Could you check a few things on this model? Use its own coordinates, in mm. A direction names the side the tool comes from. Coordinates: 2 decimals unless noted, no trailing zeros. Order: outer loops, then holes, each group sorted by start corner. A loop starts at its lowest first (then second) coordinate and runs counter-clockwise, first axis right, second up. Notation, with made-up numbers: (-28, 23) - (22, 23) arc R26 cw to (22, 47) - close; hole circle Ø3 at (-34.75, 14.25). An arc over 180 degrees is marked (long way). Answer as a JSON object with one key per item and string values. Group by question number.
(1) Imagine slicing it at D-D, the plane y = 0. Write out the boundary of the cut face in (x, z), and give its area (3 significant figures).
(2) Please list where these lines run through material, in increasing order: probe 1 along X at (y, z) = (0, 1.5); probe 2 along Y at (x, z) = (0, 8.8); probe 3 along Y at (x, z) = (0, 5.75).
(3) Which directions (+Z, -Z, +X, -X, +Y, -Y) give clear straight access to the entire face, cutting with the end or side of a thin tool? Please do faces 1 (the cylindrical face through (14, 0, 3)), 2 (the flat face through (-17.48, -3.77, 1.6)), 3 (the cylindrical face through (-14.99, 4.58, 6.12)).
(4) Imagine slicing it at A-A, the plane x = 0. Write out the boundary of the cut face in (y, z).
(5) Imagine slicing it at C-C, the plane z = 4.5. Write out the boundary of the cut face in (x, y).
(6) We'd pull the mould along X, two halves only. Please class faces 4 (the flat face through (0, 4.5, 4)), 5 (the flat face through (1, 4, 9)), 6 (the flat face through (17.48, -3.77, 1.55)): pulls with the +X half, pulls with the -X half, needs draft (parallel to the pull), parting line crosses it, or undercut.
(7) Will these pins go through, and if not, where does the flat tip stop? P1, Ø3.5, axis at x = 0, y = 0, coming from the -Z side; P2, Ø5, axis at x = -9, y = 9, coming from the -Z side; P3, Ø0.9, axis at y = 0.5, z = 2, coming from the +X side; P4, Ø9.5, axis at x = -32.5, y = 5, coming from the -Z side.
(8) Imagine slicing it at B-B, the plane z = 0.75. Write out the boundary of the cut face in (x, y).
from build123d import *

# Parameters (mm, degrees)
SKETCH1_W                    = 77.5
SKETCH1_H                    = 7
BOSS_EXTRUDE1_DEPTH          = 9
BOSS_EXTRUDE1_DEPTH_BACK     = 9
SKETCH2_W                    = 20
SKETCH2_H                    = 6.3
CUT_EXTRUDE1_DEPTH           = 8
SKETCH3_W                    = 12.5
SKETCH3_H                    = 5.85
BOSS_EXTRUDE2_DEPTH          = 8
SKETCH4_R                    = 3.04
CUT_EXTRUDE2_DEPTH           = 22
CUT_EXTRUDE2_DEPTH_BACK      = 24.5
CUT_EXTRUDE3_DEPTH           = 5
SKETCH6_R                    = 6.2
CUT_EXTRUDE4_DEPTH           = 1
MIRROR2_COPY_1_SKETCH_R      = 6.2
MIRROR2_COPY_1_DEPTH         = 1
SKETCH7_W                    = 12.5
SKETCH7_H                    = 8.5
CUT_EXTRUDE5_DEPTH           = 1
MIRROR5_COPY_1_SKETCH_W      = 12.5
MIRROR5_COPY_1_SKETCH_H      = 8.5
MIRROR5_COPY_1_DEPTH         = 1
TAP_DRILL_FOR_M2_TAP1_D      = 1.6
CUT_EXTRUDE6_DEPTH           = 27
SKETCH12_W                   = 83.830839912
SKETCH12_H                   = 36.587504352
CUT_EXTRUDE7_DEPTH           = 22
F_2_0_2_DIAMETER_HOLE1_D     = 2
F_2_0_2_DIAMETER_HOLE1_DEPTH = 30.5
F_2_0_2_DIAMETER_HOLE2_D     = 2
F_2_0_2_DIAMETER_HOLE2_DEPTH = 16
F_2_0_2_DIAMETER_HOLE2_TIP   = 0.600860619
ESQUISSE2_R                  = 3.04
BOSS_EXTRU_1_DEPTH           = 1
ESQUISSE5_R                  = 0.8
BOSS_EXTRU_3_DEPTH           = 5.85
ESQUISSE6_R                  = 0.8
BOSS_EXTRU_4_DEPTH           = 9
BOSS_EXTRUDE3_DEPTH          = 1.5
BOSS_EXTRUDE4_DEPTH          = 1
SKETCH28_R                   = 7.25
SKETCH28_R_2                 = 6.25
BOSS_EXTRUDE7_DEPTH          = 5.85
BOSS_EXTRUDE5_DEPTH          = 5.85
FILLET2_R                    = 3
CHAMFER1_SIZE                = 2.5
SKETCH27_R                   = 1
BOSS_EXTRUDE6_DEPTH          = 2
BOSS_EXTRUDE8_DEPTH          = 5.85
FILLET3_R                    = 7


with BuildPart() as part:
    # Sketch1 → Boss-Extrude1 (new body, two sides)
    with BuildSketch(Plane.XY) as boss_extrude1_sk:
        Rectangle(SKETCH1_W, SKETCH1_H)
    extrude(amount=BOSS_EXTRUDE1_DEPTH)
    extrude(boss_extrude1_sk.sketch, amount=-BOSS_EXTRUDE1_DEPTH_BACK)

    # Sketch2 → Cut-Extrude1 (cut, through all)
    with BuildSketch(Plane(origin=(0, 3.5, 0), x_dir=(1, 0, 0), z_dir=(0, 1, 0))):
        with Locations((-28.75, 0)):
            Rectangle(SKETCH2_W, SKETCH2_H)
        with Locations((28.75, 0)):
            Rectangle(SKETCH2_W, SKETCH2_H)
    extrude(amount=-CUT_EXTRUDE1_DEPTH, mode=Mode.SUBTRACT)

    # Sketch3 → Boss-Extrude2 (add)
    with BuildSketch(Plane(origin=(0, 3.5, 0), x_dir=(1, 0, 0), z_dir=(0, 1, 0))):
        with Locations((-32.5, 6.075)):
            Rectangle(SKETCH3_W, SKETCH3_H)
        with Locations((-32.5, -6.075)):
            Rectangle(SKETCH3_W, SKETCH3_H)
        with Locations((32.5, -6.075)):
            Rectangle(SKETCH3_W, SKETCH3_H)
        with Locations((32.5, 6.075)):
            Rectangle(SKETCH3_W, SKETCH3_H)
    extrude(amount=BOSS_EXTRUDE2_DEPTH)

    # Sketch4 → Cut-Extrude2 (cut, two sides)
    with BuildSketch(Plane.XY) as cut_extrude2_sk:
        with Locations((-32.5, 5)):
            Circle(SKETCH4_R)
        with Locations((32.5, 5)):
            Circle(SKETCH4_R)
    extrude(amount=CUT_EXTRUDE2_DEPTH, mode=Mode.SUBTRACT)
    extrude(cut_extrude2_sk.sketch, amount=-CUT_EXTRUDE2_DEPTH_BACK, mode=Mode.SUBTRACT)

    # Sketch5 → Cut-Extrude3 (cut)
    with BuildSketch(Plane.XY):
        Polygon((15, 3.5), (36.256888292, -2.195766051), (36.256888292, 11.5), (15, 11.5), align=None)
    extrude(amount=-CUT_EXTRUDE3_DEPTH, mode=Mode.SUBTRACT)

    # Sketch6 → Cut-Extrude4 (cut)
    with BuildSketch(Plane.XY.offset(9)):
        with Locations((32.5, 5)):
            Circle(SKETCH6_R)
    cut_extrude4 = extrude(amount=-CUT_EXTRUDE4_DEPTH, mode=Mode.SUBTRACT)

    # Mirror1: Cut-Extrude4 across plane
    add(cut_extrude4.mirror(Plane.XY), mode=Mode.SUBTRACT)

    # Mirror2: Cut-Extrude4 across plane
    add(cut_extrude4.mirror(Plane(origin=(0, 0, 0), x_dir=(0, 0, 1), z_dir=(1, 0, 0))), mode=Mode.SUBTRACT)

    # Mirror2 copy 1 sketch → Mirror2 copy 1 (cut)
    with BuildSketch(Plane(origin=(0, 0, -9), x_dir=(-1, 0, 0), z_dir=(0, 0, -1))):
        with Locations((32.5, 5)):
            Circle(MIRROR2_COPY_1_SKETCH_R)
    extrude(amount=-MIRROR2_COPY_1_DEPTH, mode=Mode.SUBTRACT)

    # Sketch7 → Cut-Extrude5 (cut)
    with BuildSketch(Plane.XY.offset(9)):
        with Locations((-32.5, 7.25)):
            Rectangle(SKETCH7_W, SKETCH7_H)
    cut_extrude5 = extrude(amount=-CUT_EXTRUDE5_DEPTH, mode=Mode.SUBTRACT)

    # Mirror3: Cut-Extrude5 across plane
    add(cut_extrude5.mirror(Plane(origin=(0, 0, 0), x_dir=(0, 0, 1), z_dir=(1, 0, 0))), mode=Mode.SUBTRACT)

    # Mirror5: Cut-Extrude5 across plane
    add(cut_extrude5.mirror(Plane.XY), mode=Mode.SUBTRACT)

    # Mirror5 copy 1 sketch → Mirror5 copy 1 (cut)
    with BuildSketch(Plane(origin=(0, 0, -9), x_dir=(-1, 0, 0), z_dir=(0, 0, -1))):
        with Locations((-32.5, 7.25)):
            Rectangle(MIRROR5_COPY_1_SKETCH_W, MIRROR5_COPY_1_SKETCH_H)
    extrude(amount=-MIRROR5_COPY_1_DEPTH, mode=Mode.SUBTRACT)

    # Tap Drill for M2 Tap1 (through all)
    with Locations(Plane.XY.offset(9)):
        with Locations((-25, 0), (0, 0), (25, 0)):
            Hole(TAP_DRILL_FOR_M2_TAP1_D / 2)

    # Sketch11 → Cut-Extrude6 (cut)
    with BuildSketch(Plane.XY.offset(9)):
        with BuildLine():
            Line((-38.75, 4.999999534), (-38.75, 21.221242017))
            Line((-38.75, 21.221242017), (-26.25, 21.221242017))
            Line((-26.25, 21.221242017), (-26.25, 4.999999534))
            ThreePointArc((-26.25, 4.999999534), (-32.5, 11.25), (-38.75, 4.999999534))
        make_face()
    cut_extrude6 = extrude(amount=-CUT_EXTRUDE6_DEPTH, mode=Mode.SUBTRACT)

    # Mirror6: Cut-Extrude6 across plane
    add(cut_extrude6.mirror(Plane(origin=(0, 0, 0), x_dir=(0, 0, 1), z_dir=(1, 0, 0))), mode=Mode.SUBTRACT)

    # Sketch12 → Cut-Extrude7 (cut)
    with BuildSketch(Plane.XY):
        Rectangle(SKETCH12_W, SKETCH12_H)
    extrude(amount=-CUT_EXTRUDE7_DEPTH, mode=Mode.SUBTRACT)

    # 2.0 _2_ Diameter Hole1
    with Locations(Plane.XY.offset(9)):
        with Locations((-15, 0)):
            Hole(F_2_0_2_DIAMETER_HOLE1_D / 2, depth=F_2_0_2_DIAMETER_HOLE1_DEPTH)

    # 2.0 _2_ Diameter Hole2
    with Locations(Plane.XY.offset(9)):
        with Locations((15, 0)):
            Hole(F_2_0_2_DIAMETER_HOLE2_D / 2, depth=F_2_0_2_DIAMETER_HOLE2_DEPTH)
            with Locations((0, 0, -(F_2_0_2_DIAMETER_HOLE2_DEPTH + F_2_0_2_DIAMETER_HOLE2_TIP / 2))):  # 118° drill point
                Cone(0, F_2_0_2_DIAMETER_HOLE2_D / 2, F_2_0_2_DIAMETER_HOLE2_TIP, mode=Mode.SUBTRACT)

    # Esquisse2 → Boss.-Extru.1 (add)
    with BuildSketch(Plane.XY.offset(8)):
        with BuildLine():
            ThreePointArc((26.6314397, 3), (31.48636147, 11.116578858), (38.7, 5))
            ThreePointArc((38.7, 5), (38.616578858, 3.98636147), (38.3685603, 3))
            Line((38.3685603, 3), (38.75, 3))
            Line((38.75, 3), (38.75, 4.999999534))
            ThreePointArc((38.75, 4.999999534), (32.5, 11.25), (26.25, 4.999999534))
            Line((26.25, 4.999999534), (26.25, 3.5))
            Line((26.25, 3.5), (26.25, 3))
            Line((26.25, 3), (26.6314397, 3))
        make_face()
        with BuildLine():
            ThreePointArc((38.3685603, 3), (38.616578858, 3.98636147), (38.7, 5))
            ThreePointArc((38.7, 5), (31.48636147, 11.116578858), (26.6314397, 3))
            ThreePointArc((26.6314397, 3), (32.5, -1.2), (38.3685603, 3))
        make_face()
        with Locations((32.5, 5)):
            Circle(ESQUISSE2_R, mode=Mode.SUBTRACT)
    boss_extru_1 = extrude(amount=BOSS_EXTRU_1_DEPTH)

    # Sym_trie1: Boss.-Extru.1 across plane
    add(boss_extru_1.mirror(Plane(origin=(0, 0, 0), x_dir=(0, 0, 1), z_dir=(1, 0, 0))))

    # Esquisse5 → Boss.-Extru.3 (add)
    with BuildSketch(Plane.XY.offset(9)):
        with Locations((-25, 0)):
            Circle(ESQUISSE5_R)
        with Locations((25, 0)):
            Circle(ESQUISSE5_R)
    extrude(amount=-BOSS_EXTRU_3_DEPTH)

    # Esquisse6 → Boss.-Extru.4 (add)
    with BuildSketch(Plane.XY.offset(9)):
        Circle(ESQUISSE6_R)
    extrude(amount=-BOSS_EXTRU_4_DEPTH)

    # Sketch22 → Boss-Extrude3 (add)
    with BuildSketch(Plane.XZ.offset(3.5)):
        Polygon((-18.75, 0), (18.75, 0), (18.75, 3.15), (38.75, 3.15), (38.75, 9), (-38.75, 9), (-38.75, 3.15), (-18.75, 3.15), align=None)
    extrude(amount=BOSS_EXTRUDE3_DEPTH)

    # Sketch23 → CSK for M2.5 Countersunk Flat Head Screw (revolve, cut)
    with BuildSketch(Plane(origin=(0, 0, 9), x_dir=(0, -1, 0), z_dir=(1, 0, 0))):
        Polygon((0, 0), (0, 9), (1.45, 9), (1.45, 2.3), (2.75, 1), (2.75, 0), align=None)
    revolve(axis=Axis((0, 0, 15.35), (0, 0, -1)), mode=Mode.SUBTRACT)

    # Sketch25 → Boss-Extrude4 (add)
    with BuildSketch(Plane(origin=(0, 3.5, 0), x_dir=(1, 0, 0), z_dir=(0, 1, 0))):
        Polygon((18.75, 0), (-18.75, 0), (-18.75, -3.15), (-26.25, -3.15), (-26.25, -9), (26.25, -9), (26.25, -3.15), (18.75, -3.15), align=None)
    extrude(amount=BOSS_EXTRUDE4_DEPTH)

    # Sketch28 → Boss-Extrude7 (add)
    with BuildSketch(Plane.XY.offset(9)):
        with Locations((-32.5, 5)):
            Circle(SKETCH28_R)
        with Locations((-32.5, 5)):
            Circle(SKETCH28_R_2, mode=Mode.SUBTRACT)
        with Locations((32.5, 5)):
            Circle(SKETCH28_R)
        with Locations((32.5, 5)):
            Circle(SKETCH28_R_2, mode=Mode.SUBTRACT)
    extrude(amount=-BOSS_EXTRUDE7_DEPTH)

    # Sketch26 → Boss-Extrude5 (add)
    with BuildSketch(Plane(origin=(0, 0, 3.15), x_dir=(-1, 0, 0), z_dir=(0, 0, -1))):
        Polygon((-29.310409021, 11.510684249), (-15, 4.5), (-25.267261929, 4.5), align=None)
        Polygon((25.267261929, 4.5), (29.310409021, 11.510684249), (15, 4.5), align=None)
    extrude(amount=-BOSS_EXTRUDE5_DEPTH)

    # Fillet2
    fillet2_edges = [part.edges().sort_by_distance(p)[0] for p in [
        (15, 4.5, 6.075),
        (-15, 4.5, 6.075),
    ]]
    fillet(fillet2_edges, radius=FILLET2_R)

    # Chamfer1
    chamfer1_edges = [part.edges().sort_by_distance(p)[0] for p in [
        (-18.75, -5, 1.575),
        (18.75, -5, 1.575),
        (18.75, 4.5, 1.575),
        (-18.75, 4.5, 1.575),
    ]]
    chamfer(chamfer1_edges, length=CHAMFER1_SIZE)

    # Sketch27 → Boss-Extrude6 (add)
    with BuildSketch(Plane.XY.offset(9)):
        with Locations((-15, 0)):
            Circle(SKETCH27_R)
        with Locations((15, 0)):
            Circle(SKETCH27_R)
    extrude(amount=-BOSS_EXTRUDE6_DEPTH)

    # Sketch29 → Boss-Extrude8 (add)
    with BuildSketch(Plane(origin=(0, 0, 3.15), x_dir=(-1, 0, 0), z_dir=(0, 0, -1))):
        Polygon((-39.75, 5), (-39.75, -5), (-38.75, -5), (-38.75, 1.325765386), align=None)
        Polygon((38.75, 1.325765386), (39.75, 5), (39.75, -5), (38.75, -5), align=None)
    extrude(amount=-BOSS_EXTRUDE8_DEPTH)

    # Fillet3
    fillet3_edges = [part.edges().sort_by_distance(p)[0] for p in [
        (39.75, -5, 6.075),
        (-39.75, -5, 6.075),
    ]]
    fillet(fillet3_edges, radius=FILLET3_R)


solid = part.part
Result set:
{
 "1": {"outline": "(-39.46, 3.15) - (-18.75, 3.15) - (-18.75, 0) - (-16, 0) - (-16, 7) - (-14, 7) - (-14, 0) - (-1.45, 0) - (-1.45, 6.7) - (-2.75, 8) - (-2.75, 9) - (-39.46, 9) - close; (1.45, 0) - (14, 0) - (14, 7) - (16, 7) - (16, 0) - (18.75, 0) - (18.75, 3.15) - (39.46, 3.15) - (39.46, 9) - (2.75, 9) - (2.75, 8) - (1.45, 6.7) - close", "area": "521 mm^2"},
 "2": {"probe 1": "x = -18.75 to -16, -14 to -1.45, 1.45 to 14, 16 to 18.75", "probe 2": "y = -5 to -2.75, 2.75 to 4.5", "probe 3": "y = -5 to -1.45, 1.45 to 4.5"},
 "3": {"face 1": "-Z", "face 2": "-Z, -X, -Y", "face 3": "+Z, -Z, +Y"},
 "4": {"outline": "(-5, 0) - (-1.45, 0) - (-1.45, 6.7) - (-2.75, 8) - (-2.75, 9) - (-5, 9) - close; (1.45, 0) - (4.5, 0) - (4.5, 9) - (2.75, 9) - (2.75, 8) - (1.45, 6.7) - close"},
 "5": {"outline": "(-39.75, 2) arc R7 ccw to (-32.75, -5) - (32.75, -5) arc R7 ccw to (39.75, 2) - (39.75, 5) arc R7.25 ccw to (29.31, 11.51) - (15.62, 4.81) arc R3 cw to (14.3, 4.5) - (-14.3, 4.5) arc R3 cw to (-15.62, 4.81) - (-29.31, 11.51) arc R7.25 ccw to (-39.75, 5) - close; hole circle Ø6.08 at (-32.5, 5); hole circle Ø2 at (-15, 0); hole circle Ø2.9 at (0, 0); hole circle Ø2 at (15, 0); hole circle Ø6.08 at (32.5, 5)"},
 "6": {"face 4": "undercut", "face 5": "needs draft", "face 6": "pulls with the +X half"},
 "7": {"P1": "stops at z = 0", "P2": "passes through", "P3": "stops at x = 18.75", "P4": "stops at z = 3.15"},
 "8": {"outline": "(-18.75, -2.5) - (-16.25, -5) - (16.25, -5) - (18.75, -2.5) - (18.75, 2) - (16.25, 4.5) - (-16.25, 4.5) - (-18.75, 2) - close; hole circle Ø2 at (-15, 0); hole circle Ø2.9 at (0, 0); hole circle Ø2 at (15, 0)"}
}
